Part model, mm, in its own coordinate system. A direction names the side the tool comes from. Coordinates: 2 decimals unless noted, no trailing zeros. Order: outer loops, then holes, each group sorted by start corner. A loop starts at its lowest first (then second) coordinate and runs counter-clockwise, first axis right, second up.
from build123d import *

# Parameters (mm, degrees)
SKETCH1_W           = 26.7
SKETCH1_H           = 70
BOSS_EXTRUDE1_DEPTH = 2
SKETCH2_W           = 2
SKETCH2_H           = 70
BOSS_EXTRUDE2_DEPTH = 12.9
SKETCH3_R           = 3.1
CUT_EXTRUDE1_DEPTH  = 77.386517135
FILLET1_R           = 1
FILLET2_R           = 1
FILLET3_R           = 1
FILLET6_R           = 1
FILLET7_R           = 1
FILLET8_R           = 1
CUT_EXTRUDE2_REACH  = 77.711
SKETCH5_W           = 12.9
SKETCH5_H           = 27
SKETCH6_W           = 12.9
SKETCH6_H           = 16
BOSS_EXTRUDE3_DEPTH = 2.25
FILLET11_R          = 1
FILLET12_R          = 1


with BuildPart() as part:
    # Sketch1 → Boss-Extrude1 (new body)
    with BuildSketch(Plane.XY):
        with Locations((13.35, 35)):
            Rectangle(SKETCH1_W, SKETCH1_H)
    extrude(amount=BOSS_EXTRUDE1_DEPTH)

    # Sketch2 → Boss-Extrude2 (add)
    with BuildSketch(Plane.XY.offset(2)):
        with Locations((1, 35)):
            Rectangle(SKETCH2_W, SKETCH2_H)
        with Locations((25.7, 35)):
            Rectangle(SKETCH2_W, SKETCH2_H)
    extrude(amount=BOSS_EXTRUDE2_DEPTH)

    # Sketch3 → Cut-Extrude1 (cut, through all)
    with BuildSketch(Plane.ZY):
        with Locations((8.2, 10)):
            Circle(SKETCH3_R)
    cut_extrude1 = extrude(amount=-CUT_EXTRUDE1_DEPTH, mode=Mode.SUBTRACT)

    # Mirror1: Cut-Extrude1 across plane
    add(cut_extrude1.mirror(Plane.ZX.offset(35)), mode=Mode.SUBTRACT)

    # Fillet1
    fillet1_edges = [part.edges().sort_by_distance(p)[0] for p in [
        (13.35, 70, 0),
    ]]
    fillet(fillet1_edges, radius=FILLET1_R)

    # Fillet2
    fillet2_edges = [part.edges().sort_by_distance(p)[0] for p in [
        (0, 34.5, 0),
        (0, 69.707106781, 0.292893219),
        (0, 70, 7.95),
    ]]
    fillet(fillet2_edges, radius=FILLET2_R)

    # Fillet3
    fillet3_edges = [part.edges().sort_by_distance(p)[0] for p in [
        (26.7, 34.5, 0),
        (26.7, 69.707106781, 0.292893219),
        (26.7, 70, 7.95),
    ]]
    fillet(fillet3_edges, radius=FILLET3_R)

    # Fillet6
    fillet6_edges = [part.edges().sort_by_distance(p)[0] for p in [
        (13.35, 0, 0),
        (0.292893219, 0, 0.292893219),
        (26.7, 0, 7.95),
        (0, 0, 7.95),
        (26.407106781, 0, 0.292893219),
    ]]
    fillet(fillet6_edges, radius=FILLET6_R)

    # Fillet7
    fillet7_edges = [part.edges().sort_by_distance(p)[0] for p in [
        (1.5, 70, 14.9),
        (0, 35, 14.9),
        (0.292893219, 69.707106781, 14.9),
        (1.5, 0, 14.9),
        (0.292893219, 0.292893219, 14.9),
    ]]
    fillet(fillet7_edges, radius=FILLET7_R)

    # Fillet8
    fillet8_edges = [part.edges().sort_by_distance(p)[0] for p in [
        (25.2, 0, 14.9),
        (25.2, 70, 14.9),
        (26.407106781, 69.707106781, 14.9),
        (26.7, 35, 14.9),
        (26.407106781, 0.292893219, 14.9),
    ]]
    fillet(fillet8_edges, radius=FILLET8_R)

    # Cut-Extrude2: up to this face of the body (flat: up to its plane)
    cut_extrude2_end = Plane(part.part.faces().sort_by_distance((26.7, 35, 7.394557998))[0])
    # Sketch5 → Cut-Extrude2 (cut, up to the picked face)
    with BuildSketch(Plane.ZY.offset(-24.7), mode=Mode.PRIVATE) as cut_extrude2_sk1:
        with Locations((8.45, 56.5)):
            Rectangle(SKETCH5_W, SKETCH5_H)
    cut_extrude2_tool1 = split(extrude(cut_extrude2_sk1.sketch, amount=-CUT_EXTRUDE2_REACH, mode=Mode.PRIVATE), bisect_by=cut_extrude2_end, keep=Keep.BOTH, mode=Mode.PRIVATE)
    # Sketch5 → Cut-Extrude2 (cut, up to the picked face)
    with BuildSketch(Plane.ZY.offset(-24.7), mode=Mode.PRIVATE) as cut_extrude2_sk2:
        with Locations((8.45, 13.5)):
            Rectangle(SKETCH5_W, SKETCH5_H)
    cut_extrude2_tool2 = split(extrude(cut_extrude2_sk2.sketch, amount=-CUT_EXTRUDE2_REACH, mode=Mode.PRIVATE), bisect_by=cut_extrude2_end, keep=Keep.BOTH, mode=Mode.PRIVATE)
    add(cut_extrude2_tool1.solids().sort_by(Axis((24.7, 56.5, 8.45), (1, 0, 0)))[0], mode=Mode.SUBTRACT)
    add(cut_extrude2_tool2.solids().sort_by(Axis((24.7, 13.5, 8.45), (1, 0, 0)))[0], mode=Mode.SUBTRACT)

    # Sketch6 → Boss-Extrude3 (add)
    with BuildSketch(Plane.ZY.offset(-24.7)):
        with Locations((8.45, 35)):
            Rectangle(SKETCH6_W, SKETCH6_H)
    extrude(amount=BOSS_EXTRUDE3_DEPTH)

    # Fillet11
    fillet11_edges = [part.edges().sort_by_distance(p)[0] for p in [
        (24.075, 27, 14.9),
        (26.407106781, 27, 14.607106781),
        (26.7, 27, 7.95),
    ]]
    fillet(fillet11_edges, radius=FILLET11_R)

    # Fillet12
    fillet12_edges = [part.edges().sort_by_distance(p)[0] for p in [
        (24.075, 43, 14.9),
        (26.407106781, 43, 14.607106781),
        (26.7, 43, 7.95),
    ]]
    fillet(fillet12_edges, radius=FILLET12_R)


solid = part.part
Q1. Cut at B-B on y = 60. Write the cut outline in (x, z), and give its area (3 significant figures).
Results list:
outline: (0, 1) arc R1 ccw to (1, 0) - (25.7, 0) arc R1 ccw to (26.7, 1) - (26.7, 2) - (2, 2) - (2, 5.1) - (0, 5.1) - close; (0, 11.3) - (2, 11.3) - (2, 14.9) - (1, 14.9) arc R1 ccw to (0, 13.9) - close
area: 66.2 mm2
Q2. Cut at D-D on y = 22. Write the cut outline in (x, z).
Results list:
outline: (0, 1) arc R1 ccw to (1, 0) - (25.7, 0) arc R1 ccw to (26.7, 1) - (26.7, 2) - (2, 2) - (2, 14.9) - (1, 14.9) arc R1 ccw to (0, 13.9) - close
Q3. Cut at C-C on x = 15.75. Write the cut outline in (y, z).
Results list:
outline: (0, 1) arc R1 ccw to (1, 0) - (69, 0) arc R1 ccw to (70, 1) - (70, 2) - (0, 2) - close
Q4. Which spindle directions (+Z, -Z, +X, -X, +Y, -Y) get a long thin tool onto all of the face, cutting with end or side? Do faces 4 (the face through (0, 35, 7)), 5 (the face through (2, 35, 8)), 6 (the face through (24, 27, 8)), 7 (the face through (24, 43, 8)). Say none if no direction does.
Results list:
face 4: +Z, -Z, -X, +Y, -Y
face 5: +Z, +Y, -Y
face 6: +Z, +X, -Y
face 7: +Z, +X, +Y
Q5. Cut at A-A on z = 8.2. Write the cut outline in (x, y).
Results list:
outline: (0, 1) arc R1 ccw to (1, 0) - (2, 0) - (2, 6.9) - (0, 6.9) - close; (0, 13.1) - (2, 13.1) - (2, 56.9) - (0, 56.9) - close; (0, 63.1) - (2, 63.1) - (2, 70) - (1, 70) arc R1 ccw to (0, 69) - close; (22.45, 27) - (25.7, 27) arc R1 ccw to (26.7, 28) - (26.7, 42) arc R1 ccw to (25.7, 43) - (22.45, 43) - close
Q6. Wall check: line 1 along Y through (x, z) = (1.1, 8.2); line 2 along X through (y, z) = (34.5, 11.25); line 3 along Z through (x, y) = (1.65, 60). Give the ranges that are in metal, low to high.
Results list:
line 1: y = 0 to 6.9, 13.1 to 56.9, 63.1 to 70
line 2: x = 0 to 2, 22.45 to 26.7
line 3: z = 0 to 5.1, 11.3 to 14.9
Q7. Mould opens along Z. For faces 1 (the face through (13, 35, 0)), 2 (the face through (0.986, 56.926, 7.796)), 3 (the face through (9.6, 0, 1.7)) say: pulls with the +Z half, pulls with the -Z half, needs draft (parallel to the pull), parting line crosses it, or undercut.
Results list:
face 1: pulls with the -Z half
face 2: undercut
face 3: needs draft
Q8. Pin check, flat tips, straight feed: pin 1 Ø1 at (x, z) = (25, 10) entering from -Y; pin 2 Ø8 at (y, z) = (60, 8.2) entering from +X; pin 3 Ø2 at (x, y) = (6.5, 11) entering from +Z. Stop position of each tip, or through.
Results list:
pin 1: stops at y = 27
pin 2: stops at x = 2
pin 3: stops at z = 2
